For this review, take the finished solid that the model builds, in its own axes (mm). A direction names the side the tool comes from. Round coordinates to 2 decimals unless told otherwise and drop trailing zeros. Write each loop counter-clockwise with the first axis right and the second up, starting at its lowest first coordinate (ties: lowest second). Pieces come first, ordered by that corner, then holes. Notation, with made-up numbers: M 82,37.5 L 130,37.5 A16 ccw 130,56.5 Z; hole C 9.5,-8.75 d7. An arc over 180 degrees is marked long. Answer in a Markdown table with one row per item.
```python
from build123d import *

# Parameters (mm, degrees)
PAD017_DEPTH              = 5
PAD020_DEPTH              = 6.25
SKETCH109_W               = 7.5
SKETCH109_H               = 1.65
PAD078_DEPTH              = 7.5
SKETCH107_W               = 2.1
SKETCH107_H               = 1.65
PAD079_DEPTH              = 7.5
SKETCH106_W               = 7.5
SKETCH106_H               = 1.65
PAD080_DEPTH              = 4.6
SKETCH108_W               = 7.5
SKETCH108_H               = 1.65
PAD081_DEPTH              = 7.5
LINEARPATTERN025_COUNT    = 2
LINEARPATTERN025_PITCH    = 3.3
CHAMFER015_SIZE           = 1
MIRROR013_PLACEMENT_ANGLE = 90


with BuildPart() as obj1:
    # Sketch034 → Pad017 (new body)
    with BuildSketch(Plane.XY):
        with BuildLine():
            Line((-1.35, -1.8), (-1.35, 6))
            ThreePointArc((0, 7.35), (-0.954594, 6.954594), (-1.35, 6))
            Line((0, 9), (0, 7.35))
            Line((-2.6, 9), (0, 9))
            Line((-2.6, -1.8), (-2.6, 9))
            Line((-3.85, -1.8), (-2.6, -1.8))
            ThreePointArc((-3.85, -1.8), (-3.439949, -2.789949), (-2.45, -3.2))
            Line((-1.35, -3.2), (-2.45, -3.2))
            Line((-1.35, -1.8), (-1.35, -3.2))
        make_face()
    extrude(amount=PAD017_DEPTH)

    # Sketch037 → Pad020 (join)
    with BuildSketch(Plane.XY):
        Polygon((-1.35, 0.2), (-1.35, 1.6), (-2.6, 1.6), (-3.85, 1.6), (-3, 0.2), (-2.6, 0.2), align=None)
    extrude(amount=PAD020_DEPTH)


with BuildPart() as obj2:
    # Mirror001: instance of _obj1
    add(obj1.part.mirror(Plane(origin=(0, 0, 0), x_dir=(0, 1, 0), z_dir=(-1, 0, 0))))


with BuildPart() as body040:
    # Fusion001 base: copy of _obj1
    add(obj1.part)

    # Fusion001: union _obj2)
    add(obj2.part)

    # Sketch109 → Pad078 (new body)
    with BuildSketch(Plane.XY):
        with Locations((1.15, 8.175)):
            Rectangle(SKETCH109_W, SKETCH109_H)
    extrude(amount=PAD078_DEPTH)

    # Sketch107 → Pad079 (join)
    with BuildSketch(Plane.XY):
        with Locations((3.85, 9.825)):
            Rectangle(SKETCH107_W, SKETCH107_H)
    pad079 = extrude(amount=PAD079_DEPTH)

    # Sketch106 → Pad080 (join)
    with BuildSketch(Plane.XY):
        with Locations((1.15, 9.825)):
            Rectangle(SKETCH106_W, SKETCH106_H)
    pad080 = extrude(amount=PAD080_DEPTH)

    # Sketch108 → Pad081 (join)
    with BuildSketch(Plane.XY):
        with Locations((1.15, 11.475)):
            Rectangle(SKETCH108_W, SKETCH108_H)
    pad081 = extrude(amount=PAD081_DEPTH)

    # LinearPattern025: Pad081, Pad080, Pad079 ×2
    with Locations(*[(0, i * LINEARPATTERN025_PITCH, 0) for i in range(1, LINEARPATTERN025_COUNT)]):
        add(pad081)
        add(pad080)
        add(pad079)

    # Chamfer015
    chamfer015_edges = [body040.edges().sort_by_distance(p)[0] for p in [
        (-2.6, 14.775, 7.5),
        (-2.6, 11.475, 7.5),
        (-2.6, 8.175, 7.5),
    ]]
    chamfer(chamfer015_edges, length=CHAMFER015_SIZE)


with BuildPart() as mirror013:
    # Mirror013: instance of Body040
    add(body040.part.mirror(Plane(origin=(0, 0, 0), x_dir=(0, -1, 0), z_dir=(1, 0, 0))))


with BuildPart() as mirror013_1:
    # Mirror013 placement: moved
    add(mirror013.part.moved(Location((2.5, 0, 5))).rotate(Axis((2.5, 0, 5), (0, -1, 0)), MIRROR013_PLACEMENT_ANGLE))


solid = mirror013_1.part
```
Q1. Mouldability with a two-part tool opening along Z and no side actions: class faces 5 (the face through (0, 1, 3.65)), 6 (the face through (-4.5, 11.5, 7.1)), 7 (the face through (0, 4, 2.4)), 8 (the face through (-2.7, 0.2, 7.6)) as +Z half, -Z half, draft (parallel to the pull), parting line (faces both ways), or undercut.
Found:
| item | result |
|---|---|
| face 5 | undercut |
| face 6 | +Z half |
| face 7 | -Z half |
| face 8 | draft |
Q2. Take a section at C-C (z = 8.25). State the section outline as (x, y) points, then the cut area to 3 significant figures.
Found:
| item | result |
|---|---|
| outline | M -3.75,0.61 L 2.5,0.61 L 2.5,1.6 L -3.75,1.6 Z; M -2.5,-2.95 L 2.5,-2.95 L 2.5,-1.8 L -2.5,-1.8 Z |
| area | 11.9 mm² |
Q3. Take a section at A-A (x = -3.5). State the section outline as (y, z) points.
Found:
| item | result |
|---|---|
| outline | M 0.2,2 L 1.6,1.15 L 1.6,3.65 L 0.2,3.65 Z; M 0.2,6.35 L 1.6,6.35 L 1.6,8.85 L 0.2,8 Z; M 7.35,0.1 L 15.6,0.1 L 15.6,7.6 L 13.95,7.6 L 13.95,2.2 L 12.3,2.2 L 12.3,7.6 L 10.65,7.6 L 10.65,2.2 L 9,2.2 L 9,7.6 L 7.35,7.6 Z |
Q4. Insertion check: P1, Ø1.5, axis at x = -0.5, y = 7.5, coming from the +Z side; P2, Ø1.5, axis at x = -4, z = 4, coming from the -Y side; P3, Ø2, axis at x = 0.5, y = -0.5, coming from the +Z side. Each pin has a flat end and moves straight along its axis. Give the tip position at first contact, or say it passes through.
Found:
| item | result |
|---|---|
| P1 | z = 7.6 |
| P2 | y = 0.2 |
| P3 | z = 8.18 |
Q5. For probe 1 along Y at (x, z) = (-4.5, 5.25); probe 2 along Z at (x, y) = (-0.25, 3); probe 3 along Z at (x, y) = (0.5, 10.5), list the stretches that pass through material, from the lowest coordinate up.
Found:
| item | result |
|---|---|
| probe 1 | 7.35 to 9, 10.65 to 12.3, 13.95 to 15.6 |
| probe 2 | 2.4 to 3.65, 6.35 to 7.6 |
| probe 3 | 0.1 to 7.6 |
Q6. Machinability: for faces 1 (the face through (0, 9, 7.6)), 2 (the face through (0, 1, 6.35)), 3 (the face through (-2.5, 5, 3)), 4 (the face through (-4, 12.3, 5)), which of the approach directions +Z, -Z, +X, -X, +Y, -Y give a long, thin tool a straight path to every point of the face, cutting with its end or side? Answer none if there is none.
Found:
| item | result |
|---|---|
| face 1 | +Z, +X, -X, +Y |
| face 2 | +X, -X, -Y |
| face 3 | +Z, -Z, -X |
| face 4 | +Z, -X |
Q7. Take a section at D-D (y = 13.5). State the section outline as (x, z) points, then the cut area to 3 significant figures.
Found:
| item | result |
|---|---|
| outline | M -5,0.1 L 2.5,0.1 L 2.5,7.6 L -2.1,7.6 L -2.1,2.2 L -5,2.2 Z |
| area | 40.6 mm² |
Q8. Take a section at B-B (y = 3). State the section outline as (x, z) points, then the cut area to 3 significant figures.
Found:
| item | result |
|---|---|
| outline | M -2.5,2.4 L 2.5,2.4 L 2.5,3.65 L -2.5,3.65 Z; M -2.5,6.35 L 2.5,6.35 L 2.5,7.6 L -2.5,7.6 Z |
| area | 12.5 mm² |
